Source: CAD feature listing. Evaluate the final solid. Frame: model axes, mm. Coordinates: 2 decimals unless noted, no trailing zeros. Order: outer loops, then holes, each group sorted by start corner. A loop starts at its lowest first (then second) coordinate and runs counter-clockwise, first axis right, second up. Notation, with made-up numbers: (24, 73) -> (45, 73) arc R24 ccw to (45, 107) -> close; hole circle Ø6 at (66.25, 15). An arc over 180 degrees is marked (long way). Write item = value, one per line. Start each with the question number.
Item 1: Mould query, pull axis X, two halves, no side actions, for faces 1 (the cylindrical face through (-39.121, -50.16, 42.416)), 2 (the flat face through (-36, -101.6, 27)), 3 (the cylindrical face through (-31.444, -50.16, 22.979)). Classes: released by +X, released by -X, zero draft, split by the parting line, or undercut.
Item 2: Ray query, line 1 along X through (y, z) = (-32, 17); line 2 along Z through (x, y) = (-14.5, -96.5); line 3 along X through (y, z) = (-83, 28.5). Return the intervals inside material, ascending. Write a range as [from, to].
Item 3: Section query A-A (y = -72.5). Output: boundary loops of the cut face in (x, z).
Item 4: Contact query for flat-ended pins moving along their axis: pin 1 (10 mm diameter, centred on x = -41, y = -17.5, fed in from +Z); pin 2 (1 mm diameter, centred on x = 19.5, y = -57, fed in from +Z); pin 3 (12 mm diameter, centred on x = 13.5, y = -55.5, fed in from +Z); pin 4 (10 mm diameter, centred on x = -29, z = 40, fed in from +Y). Output: stop coordinate, or through.
```python
from build123d import *

# Parameters (mm, degrees)
F0_R     = 38.355059125
F1_DEPTH = 101.6
F3_D     = 43.18
F4_R     = 5.08
F5_R     = 5.08


with BuildPart() as f1:
    # F0 (on Front) → F1 (new body)
    with BuildSketch(Plane.XZ):
        with Locations((-10.8512658626, 16.4939239621)):
            Circle(F0_R)
    extrude(amount=F1_DEPTH)

    # F3 (through all)
    with Locations(Plane.XZ.offset(101.6)):
        with Locations((-10.8512658626, 16.4939239621)):
            Hole(F3_D / 2)

    # F4
    f4_edges = [f1.edges().sort_by_distance(p)[0] for p in [
        (-49.206325, 0, 16.493924),
        (-32.441266, 0, 16.493924),
    ]]
    fillet(f4_edges, radius=F4_R)

    # F5
    f5_edges = [f1.edges().sort_by_distance(p)[0] for p in [
        (-49.206325, -101.6, 16.493924),
        (-32.441266, -101.6, 16.493924),
    ]]
    fillet(f5_edges, radius=F5_R)


solid = f1.part
```
Computed:
q1.face_1 = split by the parting line
q1.face_2 = zero draft
q1.face_3 = undercut
q2.line_1 = [-49.2, -32.44], [10.73, 27.5]
q2.line_2 = [-21.69, -4.79], [37.77, 54.68]
q2.line_3 = [-47.28, -28.8], [7.09, 25.58]
q3.outline = circle Ø76.71 at (-10.85, 16.49); hole circle Ø43.18 at (-10.85, 16.49)
q4.pin_1 = 45.45
q4.pin_2 = 40.58
q4.pin_3 = 50.17
q4.pin_4 = 0
